from build123d import *

# Parameters (mm, degrees)
SKETCH1_R           = 9.5
SKETCH1_W           = 80
SKETCH1_H           = 50
BOSS_EXTRUDE1_DEPTH = 3
CUT_EXTRUDE1_DEPTH  = 3
CUT_EXTRUDE3_START  = -117
CUT_EXTRUDE3_DEPTH  = 187
CUT_EXTRUDE5_DEPTH  = 3
CUT_EXTRUDE6_START  = -187
CUT_EXTRUDE6_DEPTH  = 3


with BuildPart() as part:
    # Sketch1 → Boss-Extrude1 (new body)
    with BuildSketch(Plane.XY):
        Polygon((10, 0), (190, 0), (190, 120), (9.862497021, 120), (0, 120), (0, 0), align=None)
        with Locations((45, 16.5)):
            Circle(SKETCH1_R, mode=Mode.SUBTRACT)
        with Locations((119, 90)):
            Rectangle(SKETCH1_W, SKETCH1_H, mode=Mode.SUBTRACT)
    extrude(amount=BOSS_EXTRUDE1_DEPTH)

    # Sketch3 → Cut-Extrude1 (cut)
    with BuildSketch(Plane(origin=(0, 120, 0), x_dir=(1, 0, 0), z_dir=(0, 1, 0))):
        Polygon((179.128089803, -3), (180.22, 0), (173.22, 0), (174.311910703, -3), align=None)
        Polygon((167.308089803, -3), (168.4, 0), (161.4, 0), (162.491910703, -3), align=None)
        Polygon((155.488089803, -3), (156.58, 0), (149.58, 0), (150.671910703, -3), align=None)
        Polygon((143.668089803, -3), (144.76, 0), (137.76, 0), (138.851910703, -3), align=None)
        Polygon((131.848089803, -3), (132.94, 0), (125.94, 0), (127.031910703, -3), align=None)
        Polygon((120.028089803, -3), (121.12, 0), (114.12, 0), (115.211910703, -3), align=None)
        Polygon((108.208089803, -3), (109.3, 0), (102.3, 0), (103.391910703, -3), align=None)
        Polygon((96.388089803, -3), (97.48, 0), (90.48, 0), (91.571910703, -3), align=None)
        Polygon((84.568089803, -3), (85.66, 0), (78.66, 0), (79.751910703, -3), align=None)
        Polygon((72.748089803, -3), (73.84, 0), (66.84, 0), (67.931910703, -3), align=None)
        Polygon((60.928089803, -3), (62.02, 0), (55.02, 0), (56.111910703, -3), align=None)
        Polygon((49.108089803, -3), (50.2, 0), (43.2, 0), (44.291910703, -3), align=None)
        Polygon((37.288089803, -3), (38.38, 0), (31.38, 0), (32.471910703, -3), align=None)
        Polygon((25.468089803, -3), (26.56, 0), (19.56, 0), (20.651910703, -3), align=None)
        Polygon((13.648089803, -3), (14.74, 0), (7.74, 0), (8.831910703, -3), align=None)
    extrude(amount=-CUT_EXTRUDE1_DEPTH, mode=Mode.SUBTRACT)

    # Sketch3<2> → Cut-Extrude3 (cut)
    with BuildSketch(Plane(origin=(0, 120, 0), x_dir=(1, 0, 0), z_dir=(0, 1, 0)).offset(CUT_EXTRUDE3_START)):
        Polygon((179.128089803, -3), (180.22, 0), (173.22, 0), (174.311910703, -3), align=None)
        Polygon((167.308089803, -3), (168.4, 0), (161.4, 0), (162.491910703, -3), align=None)
        Polygon((155.488089803, -3), (156.58, 0), (149.58, 0), (150.671910703, -3), align=None)
        Polygon((143.668089803, -3), (144.76, 0), (137.76, 0), (138.851910703, -3), align=None)
        Polygon((131.848089803, -3), (132.94, 0), (125.94, 0), (127.031910703, -3), align=None)
        Polygon((120.028089803, -3), (121.12, 0), (114.12, 0), (115.211910703, -3), align=None)
        Polygon((108.208089803, -3), (109.3, 0), (102.3, 0), (103.391910703, -3), align=None)
        Polygon((96.388089803, -3), (97.48, 0), (90.48, 0), (91.571910703, -3), align=None)
        Polygon((84.568089803, -3), (85.66, 0), (78.66, 0), (79.751910703, -3), align=None)
        Polygon((72.748089803, -3), (73.84, 0), (66.84, 0), (67.931910703, -3), align=None)
        Polygon((60.928089803, -3), (62.02, 0), (55.02, 0), (56.111910703, -3), align=None)
        Polygon((49.108089803, -3), (50.2, 0), (43.2, 0), (44.291910703, -3), align=None)
        Polygon((37.288089803, -3), (38.38, 0), (31.38, 0), (32.471910703, -3), align=None)
        Polygon((25.468089803, -3), (26.56, 0), (19.56, 0), (20.651910703, -3), align=None)
        Polygon((13.648089803, -3), (14.74, 0), (7.74, 0), (8.831910703, -3), align=None)
    extrude(amount=-CUT_EXTRUDE3_DEPTH, mode=Mode.SUBTRACT)

    # Sketch6 → Cut-Extrude5 (cut)
    with BuildSketch(Plane.ZY):
        Polygon((0, 104.7919109), (3, 103.7), (3, 110.7), (0, 109.60809), align=None)
        Polygon((0, 92.9919109), (3, 91.9), (3, 98.9), (0, 97.80809), align=None)
        Polygon((0, 81.1919109), (3, 80.1), (3, 87.1), (0, 86.00809), align=None)
        Polygon((0, 69.3919109), (3, 68.3), (3, 75.3), (0, 74.20809), align=None)
        Polygon((0, 57.5919109), (3, 56.5), (3, 63.5), (0, 62.40809), align=None)
        Polygon((0, 45.7919109), (3, 44.7), (3, 51.7), (0, 50.60809), align=None)
        Polygon((0, 33.9919109), (3, 32.9), (3, 39.9), (0, 38.80809), align=None)
        Polygon((0, 22.1919109), (3, 21.1), (3, 28.1), (0, 27.00809), align=None)
        Polygon((0, 10.3919109), (3, 9.3), (3, 16.3), (0, 15.20809), align=None)
    extrude(amount=-CUT_EXTRUDE5_DEPTH, mode=Mode.SUBTRACT)

    # Sketch6<3> → Cut-Extrude6 (cut)
    with BuildSketch(Plane.ZY.offset(CUT_EXTRUDE6_START)):
        Polygon((0, 104.7919109), (3, 103.7), (3, 110.7), (0, 109.60809), align=None)
        Polygon((0, 92.9919109), (3, 91.9), (3, 98.9), (0, 97.80809), align=None)
        Polygon((0, 81.1919109), (3, 80.1), (3, 87.1), (0, 86.00809), align=None)
        Polygon((0, 69.3919109), (3, 68.3), (3, 75.3), (0, 74.20809), align=None)
        Polygon((0, 57.5919109), (3, 56.5), (3, 63.5), (0, 62.40809), align=None)
        Polygon((0, 45.7919109), (3, 44.7), (3, 51.7), (0, 50.60809), align=None)
        Polygon((0, 33.9919109), (3, 32.9), (3, 39.9), (0, 38.80809), align=None)
        Polygon((0, 22.1919109), (3, 21.1), (3, 28.1), (0, 27.00809), align=None)
        Polygon((0, 10.3919109), (3, 9.3), (3, 16.3), (0, 15.20809), align=None)
    extrude(amount=-CUT_EXTRUDE6_DEPTH, mode=Mode.SUBTRACT)


solid = part.part
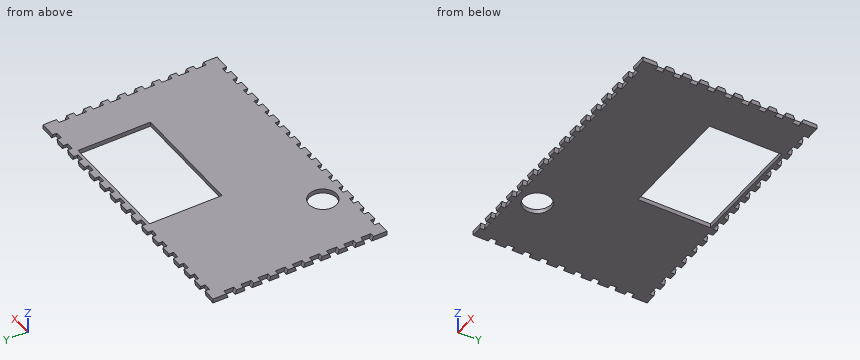
Part model, mm, in its own coordinate system. Give positions to 0.01 mm unless a question says otherwise; leave off trailing zeros. Loops run counter-clockwise (first coordinate to the right, second up) from the corner with the lowest first, then second, coordinate; pieces in that order, holes last. Notation, with made-up numbers: M 2,-21 L 31,-21 A13 cw 31,-3 Z; hole C 24.25,36 d11. An arc over 180 degrees is marked long. Put each result on its own line as item: value. Start each with the question number.
1) Probe probe 1 along Y at (x, z) = (45, 0.8); probe 2 along X at (y, z) = (65.5, 2.65); probe 3 along Y at (x, z) = (93.5, 1.5). List the from-to ranges inside material, lowest first.
2) Saw through at A-A (y = 96). List the corners of the cut face in (x, z), then the cut area to 3 significant figures.
3) Flat gauge pins, fed straight in: pin 1 (0.9 mm diameter, centred on y = 82, z = 2, fed in from -X); pin 2 (0.9 mm diameter, centred on y = 72, z = 1.5, fed in from +X); pin 3 (1.5 mm diameter, centred on x = 118, z = 2, fed in from +Y). Where does each tip first touch, or does it go through?
4) Saw through at B-B (z = 0.5). State how many separate pieces and enclosed holes the cut face has, then the cut area to 3 significant figures.
Numbers:
1. probe 1: 3 to 7, 26 to 117
1. probe 2: 0 to 79, 159 to 190
1. probe 3: 3 to 65, 115 to 117
2. outline: M 3,0 L 79,0 L 79,3 L 3,3 Z; M 159,0 L 187,0 L 187,3 L 159,3 Z
2. area: 312 mm^2
3. pin 1: x = 3
3. pin 2: x = 187
3. pin 3: y = 117
4. separate pieces: 1
4. enclosed holes: 2
4. area: 17,600 mm^2
